from build123d import *

# Parameters (mm, degrees)
F0_W           = 8
F0_H           = 80
F0_R           = 3.225
F1_DEPTH       = 10
F3_D           = 4
F3_CBORE_D     = 7
F3_CBORE_DEPTH = 4
F4_R           = 3
F2_R           = 3.225
F5_DEPTH       = 6
F6_D           = 4


with BuildPart() as f1:
    # F0 (on Top) → F1 (new body)
    with BuildSketch(Plane.XY):
        Rectangle(F0_W, F0_H)
        with Locations((0, -15)):
            Circle(F0_R, mode=Mode.SUBTRACT)
        with Locations((0, -5)):
            Circle(F0_R, mode=Mode.SUBTRACT)
        with Locations((0, 5)):
            Circle(F0_R, mode=Mode.SUBTRACT)
        with Locations((0, 15)):
            Circle(F0_R, mode=Mode.SUBTRACT)
        with Locations((0, 5)):
            Circle(F0_R)
        with Locations((0, -5)):
            Circle(F0_R)
        with Locations((0, 15)):
            Circle(F0_R)
        with Locations((0, -15)):
            Circle(F0_R)
    extrude(amount=F1_DEPTH)

    # F3 (through all)
    with Locations(Plane.XY.offset(10)):
        with Locations((0, 28.575), (0, -28.575)):
            CounterBoreHole(F3_D / 2, F3_CBORE_D / 2, F3_CBORE_DEPTH)

    # F4
    f4_edges = [f1.edges().sort_by_distance(p)[0] for p in [
        (-4, 40, 5),
        (4, 40, 5),
        (-4, -40, 5),
        (4, -40, 5),
    ]]
    fillet(f4_edges, radius=F4_R)

    # F2 (on face) → F5 (cut)
    with BuildSketch(Plane.XY.offset(10)):
        with Locations((0, -5)):
            Circle(F2_R)
        with Locations((0, 5)):
            Circle(F2_R)
        with Locations((0, 15)):
            Circle(F2_R)
        with Locations((0, -15)):
            Circle(F2_R)
    extrude(amount=-F5_DEPTH, mode=Mode.SUBTRACT)

    # F6 (through all)
    with Locations(Plane(origin=(0, 0, 0), x_dir=(1, 0, 0), z_dir=(0, 0, -1))):
        with Locations((0, 15), (0, 5), (0, -5), (0, -15)):
            Hole(F6_D / 2)


solid = f1.part
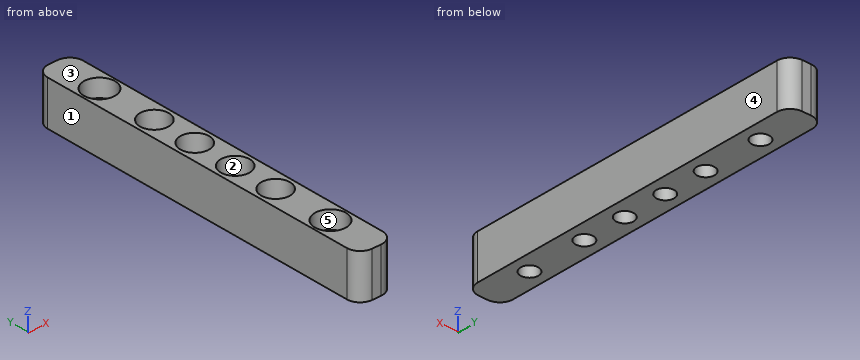
Verification items for the finished model (mm, model axes). Face numbers are marked on the shaded views. A direction names the side the tool comes from. Coordinates: 2 decimals unless noted, no trailing zeros. Loops run counter-clockwise (first coordinate to the right, second up) from the corner with the lowest first, then second, coordinate; pieces in that order, holes last. Notation, with made-up numbers: M 14,63 L 58,63 A25 cw 58,87 Z; hole C -38,88 d1. An arc over 180 degrees is marked long. One line per item, written item: value.
1. Material ranges on line 1 along X through (y, z) = (-15, 0.95); line 2 along X through (y, z) = (26, 7); line 3 along Z through (x, y) = (3, -16), recorded low to high. Write a range as from..to.
Answers follow:
line 1: -4..-2, 2..4
line 2: -4..-2.37, 2.37..4
line 3: 0..4
2. Section check B-B on z = 8. Record the cut outline in (x, y) (3 decimals), plus the area to 3 significant figures.
Answers follow:
outline: M -4,-37 A3 ccw -1,-40 L 1,-40 A3 ccw 4,-37 L 4,37 A3 ccw 1,40 L -1,40 A3 ccw -4,37 Z; hole C 0,-28.575 d7; hole C 0,28.575 d7; hole C 0,-15 d6.45; hole C 0,-5 d6.45; hole C 0,5 d6.45; hole C 0,15 d6.45
area: 425 mm^2
3. Set-up check for the marked faces 4 and 5: record each of +Z, -Z, +X, -X, +Y, -Y from which the full face is reachable in a straight line by a thin tool's end or side.
Answers follow:
face 4: +Z, -Z, +X, +Y, -Y
face 5: +Z
4. Section check A-A on y = 5. Record the cut outline in (x, z) (3 decimals).
Answers follow:
outline: M -4,0 L -2,0 L -2,4 L -3.225,4 L -3.225,10 L -4,10 Z; M 2,0 L 4,0 L 4,10 L 3.225,10 L 3.225,4 L 2,4 Z
5. Mould release check, pull along X, two halves, no side actions. Record for the marked faces 1, 2 and 3: pulls with the +X half, pulls with the -X half, needs draft (parallel to the pull), parting line crosses it, or undercut.
Answers follow:
face 1: pulls with the -X half
face 2: undercut
face 3: needs draft
